Geometry: final body of the model. Coordinates: model frame, mm. A direction names the side the tool comes from. Give positions to 0.01 mm unless a question says otherwise; leave off trailing zeros. Order: outer loops, then holes, each group sorted by start corner. A loop starts at its lowest first (then second) coordinate and runs counter-clockwise, first axis right, second up. Notation, with made-up numbers: (50, 18) - (82, 18) arc R22 cw to (82, 27) - close; hole circle Ø6 at (28.25, -30). An arc over 180 degrees is marked (long way). One line per item, written item: value.
```python
from build123d import *

# Parameters (mm, degrees)
EXTRUDE_1_DEPTH = 5


with BuildPart() as part:
    # 草图1 → 凸台-拉伸1 (new body)
    with BuildSketch(Plane.XY):
        with BuildLine():
            Line((-80.978778084, -25), (-47.25, -25))
            Line((-47.25, -25), (-47.25, -40))
            Line((-47.25, -40), (-48.65, -40))
            Line((-48.65, -40), (-48.65, -43.5))
            Line((-48.65, -43.5), (-47.25, -43.5))
            Line((-47.25, -43.5), (-47.25, -50))
            Line((-47.25, -50), (-42.75, -50))
            Line((-42.75, -50), (-42.75, -43.5))
            Line((-42.75, -43.5), (-41.35, -43.5))
            Line((-41.35, -43.5), (-41.35, -40))
            Line((-41.35, -40), (-42.75, -40))
            Line((-42.75, -40), (-42.75, -25))
            Line((-42.75, -25), (42.75, -25))
            Line((42.75, -25), (42.75, -40))
            Line((42.75, -40), (41.35, -40))
            Line((41.35, -40), (41.35, -43.5))
            Line((41.35, -43.5), (42.75, -43.5))
            Line((42.75, -43.5), (42.75, -50))
            Line((42.75, -50), (47.25, -50))
            Line((47.25, -50), (47.25, -43.5))
            Line((47.25, -43.5), (48.65, -43.5))
            Line((48.65, -43.5), (48.65, -40))
            Line((48.65, -40), (47.25, -40))
            Line((47.25, -40), (47.25, -25))
            Line((47.25, -25), (80.978778084, -25))
            ThreePointArc((80.978778084, -25), (61.76714503, -58.029150389), (30, -79.262617292))
            Line((30, -79.262617292), (30, -49.262617292))
            Line((30, -49.262617292), (-30, -49.262617292))
            Line((-30, -49.262617292), (-30, -79.262617292))
            ThreePointArc((-30, -79.262617292), (-61.76714503, -58.029150389), (-80.978778084, -25))
        make_face()
    extrude(amount=EXTRUDE_1_DEPTH)


solid = part.part
```
1) Section A-A, the plane y = -52. Return loops of the section in (x, z), then the cut area to 3 significant figures.
Answers below:
outline: (-66.92, 0) - (-30, 0) - (-30, 5) - (-66.92, 5) - close; (30, 0) - (66.92, 0) - (66.92, 5) - (30, 5) - close
area: 369 mm^2
2) Set-up query: faces 1 (the face through (30, -64, 2)), 2 (the face through (-42.75, -47, 2)), 3 (the face through (64, -25, 2)). Return all of +Z, -Z, +X, -X, +Y, -Y with unobstructed straight access to the full face (end or side cutting, diameter ignored); none if empty.
Answers below:
face 1: +Z, -Z, -Y
face 2: +Z, -Z, +Y
face 3: +Z, -Z, +X, -X, +Y
3) Material intervals for line 1 along X through (y, z) = (-29.5, 0.95); line 2 along Y through (x, z) = (-10, 1.55); line 3 along X through (y, z) = (-38, 2.5), sorted ascending.
Answers below:
line 1: -79.45 to -47.25, -42.75 to 42.75, 47.25 to 79.45
line 2: -49.26 to -25
line 3: -75.75 to -47.25, -42.75 to 42.75, 47.25 to 75.75
4) First-contact query: pin 1 (1.8 mm diameter, centred on y = -41, z = 3.5, fed in from -X); pin 2 (1.5 mm diameter, centred on x = -47.5, z = 3.5, fed in from -Y); pin 3 (1.5 mm diameter, centred on y = -70, z = 2.5, fed in from +X). Flat tips, straight axial feed; report the tip coordinate or a pass-through.
Answers below:
pin 1: x = -74.66
pin 2: y = -70.69
pin 3: x = 48.86
5) Mould query, pull axis Y, two halves, no side actions, for faces 4 (the face through (-48.65, -42, 2)), 5 (the face through (1, -46, 5)), 6 (the face through (48.65, -42, 2)), 7 (the face through (62.14, -57.63, 2.46)). Classes: released by +Y, released by -Y, zero draft, split by the parting line, or undercut.
Answers below:
face 4: undercut
face 5: zero draft
face 6: undercut
face 7: released by -Y
6) Section D-D, the plane x = -16. Return loops of the section in (y, z), then the cut area to 3 significant figures.
Answers below:
outline: (-49.26, 0) - (-25, 0) - (-25, 5) - (-49.26, 5) - close
area: 121 mm^2
7) Section C-C, the plane y = -34. Return loops of the section in (x, z).
Answers below:
outline: (-77.63, 0) - (-47.25, 0) - (-47.25, 5) - (-77.63, 5) - close; (-42.75, 0) - (42.75, 0) - (42.75, 5) - (-42.75, 5) - close; (47.25, 0) - (77.63, 0) - (77.63, 5) - (47.25, 5) - close
